Autodesk Inventor part; units mm, degrees
ref_plane "YZ Plane" through (0, 0, 0) normal (1, 0, 0) x (0, 1, 0)
ref_plane "XZ Plane" through (0, 0, 0) normal (0, 1, 0) x (-1, 0, 0)
ref_plane "XY Plane" through (0, 0, 0) normal (0, 0, 1) x (1, 0, 0)
sketch "Sketch1" plane through (0, 0, 0) normal (0, 0, 1) x (1, 0, 0)
  line L0 (-240, 35) -> (240, 35)
  line L1 (240, 35) -> (240, -35)
  line L2 (240, -35) -> (-240, -35)
  line L3 (-240, -35) -> (-240, 35)
  line L4 (-240, 35) -> (240, -35) construction
  line L5 (240, 35) -> (-240, -35) construction
  point P0 (0, 0)
  dimension "d0" = 70
  dimension "d1" = 480
extrude "Extrusion1" add sketch "Sketch1" along normal mid plane 3
sketch "Sketch2" plane through (0, 0, 1.5) normal (0, 0, 1) x (1, 0, 0)
  line L0 (-225.0001, 20) -> (225.0001, 20)
  line L1 (225.0001, 20) -> (225.0001, -25)
  line L2 (225.0001, -25) -> (-225.0001, -25)
  line L3 (-225.0001, -25) -> (-225.0001, 20)
  line L4 (240, 35) -> (-240, 35)
  line L5 (-240, -35) -> (240, -35)
  line L6 (-225.0001, -5) -> (225.0001, -5)
  line L7 (-240, 35) -> (-240, -35)
  point P0 (0, 0)
  point P1 (0, 20)
  point P2 (-205.0001, 20)
  point P3 (-205.0001, -25)
  point P4 (205.0001, 20)
  point P5 (205.0001, -25)
  point P6 (0, 20)
  point P7 (0, -25)
  point P8 (-205.0001, -5)
  point P9 (0, -5)
  point P10 (205.0001, -5)
  dimension "d5" = 15
  dimension "d19" = 20
  dimension "d20" = 20
  dimension "d21" = 10
  dimension "d22" = 20
  dimension "d23" = 14.9999
hole "Hole1" at (-205.0001, 20, 1.5) at (-205.0001, -25, 1.5) at (205.0001, 20, 1.5) at (205.0001, -25, 1.5) at (0, 20, 1.5) at (0, -25, 1.5) at (-205.0001, -5, 1.5) at (0, -5, 1.5) at (205.0001, -5, 1.5) direction (0, 0, -1) diameter 4.5 end through all countersink diameter 9.4 countersink angle 90
fillet "Fillet1" radius 2 4 edges at (240, -35, 0) (240, 35, 0) (-240, -35, 0) (-240, 35, 0)
properties part number "PBLMK-041-2" material "Aluminum"
CAD build for the part. Positions are in the model's coordinates, mm. Coordinates: 2 decimals unless noted, no trailing zeros. Use CSV: the item, a comma, the result in double quotes. Start each with the question number.
Q1. Drop flat-ended pins along their axis: P1, Ø2.5, axis at x = 205, y = 20, coming from the -Z side; P2, Ø5, axis at x = 0, y = -5, coming from the +Z side; P3, Ø6, axis at x = -205, y = -5, coming from the +Z side. Give the stop position or say it passes through.
Q2. Probe probe 1 along Y at (x, z) = (0, -1.15); probe 2 along X at (y, z) = (20, -1.25); probe 3 along X at (y, z) = (20, -0.3). List the from-to ranges inside material, lowest first. Write a range as from..to.
Q3. Two-plate mould, pull along X, no slides. Class faces 1 (the conical face through (-2.13, -26.11, -0.8)), 2 (the flat face through (-3, 0, -1.5)): +X half, -X half, draft (parallel to the pull), parting line (faces both ways), or undercut.
Here are the results:
1,P1,"through"
1,P2,"z = -0.7"
1,P3,"z = -0.2"
2,probe 1,"-35..-27.25, -22.75..-7.25, -2.75..17.75, 22.25..35"
2,probe 2,"-240..-207.25, -202.75..-2.25, 2.25..202.75, 207.25..240"
2,probe 3,"-240..-207.9, -202.1..-2.9, 2.9..202.1, 207.9..240"
3,face 1,"undercut"
3,face 2,"draft"
